Read the model definition and answer for the solid it produces. Units are mm, in the model's axes. A direction names the side the tool comes from. Coordinates: 2 decimals unless noted, no trailing zeros. Loops run counter-clockwise (first coordinate to the right, second up) from the corner with the lowest first, then second, coordinate; pieces in that order, holes last. Notation, with made-up numbers: M 16,64 L 71,64 A17 cw 71,74 Z; hole C 58.5,79.5 d11. An arc over 180 degrees is marked long. One line per item, written item: value. Start each with the question number.
1. Determine the mould class of faces 6 (the face through (19, 16, -40)), 7 (the face through (10, 35, -10)), 8 (the face through (15, 16, 0)), 9 (the face through (10, 40, -5)) for opening direction Z: +Z half, -Z half, draft (parallel to the pull), parting line (faces both ways), or undercut.
2. For faces 1 (the face through (10, 35, -30)), 2 (the face through (0, 15, -20)), 3 (the face through (40, 5, -10)), 4 (the face through (35, 10, -24)), 5 (the face through (70, 20, -30)), determine the directions among +Z, -Z, +X, -X, +Y, -Y from which every point of the face is accessible in a straight line to the end or side of a thin tool.
3. Consider probe 1 along Z at (x, y) = (13.5, 30.5); probe 2 along X at (y, z) = (27, -31); probe 3 along X at (y, z) = (30, -9.5). Determine where each line is inside the solid, lowest interval first.
4. Flat-ended cylindrical pins translate along their axes: pin 1 (8 mm diameter, centred on x = 29.5, z = -35.5, fed in from +Y); pin 2 (5 mm diameter, centred on y = 18.5, z = -15.5, fed in from +X); pin 3 (3 mm diameter, centred on y = 7, z = -13, fed in from +X). Find the tip coordinate at first contact, or state that the pin passes through.
5. The part is cut by section B-B (x = 15.5). Write down the section's boundary in (y, z).
6. The part is cut by section C-C (z = -8). Write down the section's boundary in (x, y), then the cut area to 3 significant figures.
7. The part is cut by section D-D (x = 57.5). Write down the section's boundary in (y, z), then the cut area to 3 significant figures.
8. The part is cut by section A-A (z = -31). Write down the section's boundary in (x, y).
```python
from build123d import *

# Parameters (mm, degrees)
SKETCH_1_W          = 70
SKETCH_1_H          = 40
EXTRUDE_1_DEPTH     = 40
SKETCH_2_W          = 40
SKETCH_2_H          = 30
CUT_EXTRUDE_1_DEPTH = 40
SKETCH_3_W          = 30
SKETCH_3_H          = 20
CUT_EXTRUDE_2_DEPTH = 40
CUT_EXTRUDE_3_DEPTH = 40


with BuildPart() as part:
    # 스케치1 → 보스-돌출1 (new body)
    with BuildSketch(Plane.XY):
        with Locations((35, 20)):
            Rectangle(SKETCH_1_W, SKETCH_1_H)
    extrude(amount=-EXTRUDE_1_DEPTH)

    # 스케치2 → 컷-돌출1 (cut)
    with BuildSketch(Plane.XY):
        with Locations((40, 25)):
            Rectangle(SKETCH_2_W, SKETCH_2_H)
    extrude(amount=-CUT_EXTRUDE_1_DEPTH, mode=Mode.SUBTRACT)

    # 스케치3 → 컷-돌출2 (cut)
    with BuildSketch(Plane(origin=(0, 40, 0), x_dir=(1, 0, 0), z_dir=(0, 1, 0))):
        with Locations((55, 10)):
            Rectangle(SKETCH_3_W, SKETCH_3_H)
    extrude(amount=-CUT_EXTRUDE_2_DEPTH, mode=Mode.SUBTRACT)

    # 스케치4 → 컷-돌출3 (cut)
    with BuildSketch(Plane.ZY):
        with BuildLine():
            Line((-30, 40), (-30, 30))
            ThreePointArc((-30, 30), (-20, 20), (-10, 30))
            Line((-10, 30), (-10, 40))
            Line((-10, 40), (-30, 40))
        make_face()
    extrude(amount=-CUT_EXTRUDE_3_DEPTH, mode=Mode.SUBTRACT)


solid = part.part
```
Answer block:
1. face 6: -Z half
1. face 7: undercut
1. face 8: +Z half
1. face 9: draft
2. face 1: -X, +Y
2. face 2: +Z, -Z, -X, +Y, -Y
2. face 3: +Z, +X, +Y, -Y
2. face 4: +Z, -Z, +Y
2. face 5: +Z, -Z, +X, +Y, -Y
3. probe 1: z = -40 to -30, -10 to 0
3. probe 2: x = 0 to 20, 60 to 70
3. probe 3: x = 0 to 20
4. pin 1: stops at y = 10
4. pin 2: stops at x = 20
4. pin 3: stops at x = 40
5. outline: M 0,-40 L 40,-40 L 40,-30 L 30,-30 A10 cw 30,-10 L 40,-10 L 40,0 L 0,0 Z
6. outline: M 0,0 L 40,0 L 40,10 L 20,10 L 20,40 L 0,40 Z
6. area: 1,000 mm2
7. outline: M 0,-40 L 10,-40 L 10,-20 L 0,-20 Z
7. area: 200 mm2
8. outline: M 0,0 L 70,0 L 70,40 L 60,40 L 60,10 L 20,10 L 20,40 L 0,40 Z
